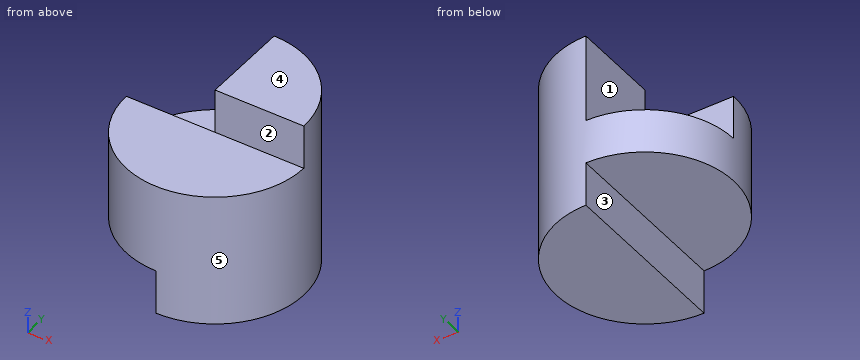
from build123d import *

# Parameters (mm, degrees)
SKETCH1_R               = 20
BOSS_EXTRUDE1_DEPTH     = 40
SKETCH2_W               = 20
SKETCH2_H               = 10
CUT_EXTRUDE1_DEPTH      = 40
CUT_EXTRUDE1_DEPTH_BACK = 40
SKETCH3_W               = 10
SKETCH3_H               = 20
CUT_EXTRUDE2_DEPTH      = 40
CUT_EXTRUDE3_DEPTH      = 10


with BuildPart() as part:
    # Sketch1 → Boss-Extrude1 (new body)
    with BuildSketch(Plane.XY):
        Circle(SKETCH1_R)
    extrude(amount=BOSS_EXTRUDE1_DEPTH)

    # Sketch2 → Cut-Extrude1 (cut, two sides)
    with BuildSketch(Plane(origin=(0, 0, 0), x_dir=(1, 0, 0), z_dir=(0, 1, 0))) as cut_extrude1_sk:
        with Locations((-10, -5)):
            Rectangle(SKETCH2_W, SKETCH2_H)
        with Locations((-10, -35)):
            Rectangle(SKETCH2_W, SKETCH2_H)
    extrude(amount=CUT_EXTRUDE1_DEPTH, mode=Mode.SUBTRACT)
    extrude(cut_extrude1_sk.sketch, amount=-CUT_EXTRUDE1_DEPTH_BACK, mode=Mode.SUBTRACT)

    # Sketch3 → Cut-Extrude2 (cut)
    with BuildSketch(Plane.ZY):
        with Locations((35, -10)):
            Rectangle(SKETCH3_W, SKETCH3_H)
    extrude(amount=-CUT_EXTRUDE2_DEPTH, mode=Mode.SUBTRACT)

    # Sketch4 → Cut-Extrude3 (cut)
    with BuildSketch(Plane.XY.offset(30)):
        with BuildLine():
            Line((-20, 0), (0, 0))
            Line((0, 0), (0, 20))
            ThreePointArc((0, 20), (-14.142135624, 14.142135624), (-20, 0))
        make_face()
    extrude(amount=-CUT_EXTRUDE3_DEPTH, mode=Mode.SUBTRACT)


solid = part.part
Could you check a few things on this model? Use its own coordinates, in mm. Face numbers are marked on the shaded views. A direction names the side the tool comes from. Give positions to 0.01 mm unless a question says otherwise; leave off trailing zeros. Write each loop counter-clockwise with the first axis right and the second up, starting at its lowest first coordinate (ties: lowest second). Pieces come first, ordered by that corner, then holes. Notation, with made-up numbers: (57.5, -27.5) -> (103.5, -27.5) arc R16 cw to (103.5, -8.5) -> close; hole circle Ø2 at (86.25, 0). An arc over 180 degrees is marked (long way). Write each question's results on one line, items separated by ' | '. Start each with the question number.
Q1. Suppose I cut it at C-C, the plane x = -14. List the corners of the cut face in (y, z) for me, and give its area (3 significant figures).
Q2. I need wall thicknesses on probe 1 along Z at (x, y) = (10, -11); probe 2 along Z at (x, y) = (-2.5, 18.5); probe 3 along Y at (x, z) = (0.5, 17). Which ranges of each line are inside material? Lowest first, please.
Q3. Suppose I cut it at A-A, the plane y = 1. List the corners of the cut face in (x, z) for me.
Q4. Which directions (+Z, -Z, +X, -X, +Y, -Y) give clear straight access to the entire face, cutting with the end or side of a thin tool? Please do the marked faces 1, 2, 3, 4 and 5.
Q5. I'm going to push flat-ended pins straight in: pin 1 Ø6 at (y, z) = (10.5, 33.5) entering from -X; pin 2 Ø6 at (x, y) = (-13, 10) entering from +Z; pin 3 Ø6 at (x, z) = (8, 33.5) entering from +Y. Where does each tip first touch, or does it pass through?
Q6. Suppose I cut it at D-D, the plane y = -6. List the corners of the cut face in (x, z) for me.
Q7. Suppose I cut it at B-B, the plane z = 32.5. List the corners of the cut face in (x, y) for me.
Outcome:
1) outline: (-14.28, 10) -> (14.28, 10) -> (14.28, 20) -> (0, 20) -> (0, 30) -> (-14.28, 30) -> close | area: 428 mm2
2) probe 1: 0 to 30 | probe 2: 10 to 20 | probe 3: -19.99 to 19.99
3) outline: (-19.97, 10) -> (0, 10) -> (0, 0) -> (19.97, 0) -> (19.97, 40) -> (0, 40) -> (0, 20) -> (-19.97, 20) -> close
4) face 1: +Z, -X, +Y | face 2: +Z, +X, -X, -Y | face 3: -Z, -X, +Y, -Y | face 4: +Z, +X, -X, +Y, -Y | face 5: +Z, -Z
5) pin 1: x = 0 | pin 2: z = 20 | pin 3: y = 19.36
6) outline: (-19.08, 10) -> (0, 10) -> (0, 0) -> (19.08, 0) -> (19.08, 30) -> (-19.08, 30) -> close
7) outline: (0, 0) -> (20, 0) arc R20 ccw to (0, 20) -> close
